Job drawing, mm, ordinate dimensions from the low corner. One solid piece. A direction names the side the tool comes from. Give positions to 0.01 mm unless a question says otherwise; leave off trailing zeros. Order: outer loops, then holes, each group sorted by start corner. A loop starts at its lowest first (then second) coordinate and runs counter-clockwise, first axis right, second up. Notation, with made-up numbers: (78.5, 26.25) - (90.5, 26.25) arc R12 ccw to (90.5, 33.25) - close; hole circle Ø10 at (89, 18.25). An arc over 180 degrees is marked (long way). Write each question's results on one line, items separated by ' | '. Start each with the question number.
1) Cut at C-C on y = 10. List the corners of the cut face in (x, z).
2) Drop flat-ended pins along their axis: pin 1 Ø7 at (x, y) = (10, 70) entering from -Z; pin 2 Ø17.5 at (y, z) = (18.5, 29) entering from -X; pin 3 Ø1.2 at (x, z) = (11.5, 3) entering from -Y; pin 4 Ø1.2 at (x, z) = (11, 1.5) entering from +Y. Give the stop position or say it passes through.
3) Cut at A-A on z = 29. List the corners of the cut face in (x, y), plus the area to 3 significant figures.
4) Tool access for the marked faces 1 and 2: list every direction of +Z, -Z, +X, -X, +Y, -Y with a clear straight run to the whole face (end or side of a thin tool).
5) Drill centre lines: line 1 along Z through (x, y) = (13, 130); line 2 along Y through (x, z) = (10, 7.5); line 3 along Y through (x, z) = (10.25, 15). Where is each one in solid material? Low to high. Write a range as from..to.
6) Cut at B-B on y = 70. List the corners of the cut face in (x, z).
7) Cut at D-D on y = 119.5. List the corners of the cut face in (x, z).
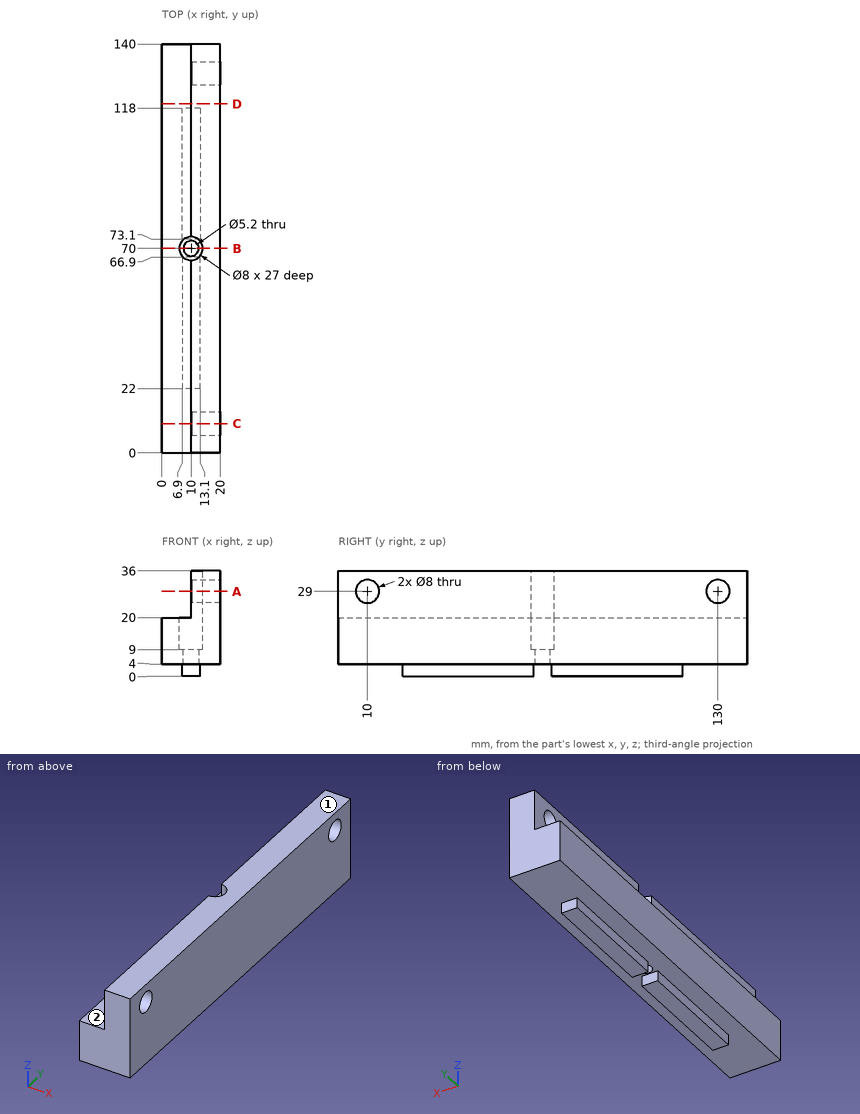
Results:
1) outline: (0, 4) - (20, 4) - (20, 25) - (10, 25) - (10, 20) - (0, 20) - close; (10, 33) - (20, 33) - (20, 36) - (10, 36) - close
2) pin 1: z = 0 | pin 2: x = 10 | pin 3: y = 22 | pin 4: y = 118
3) outline: (10, 0) - (20, 0) - (20, 6) - (10, 6) - close; (10, 14) - (20, 14) - (20, 126) - (10, 126) - (10, 74) arc R4 cw to (10, 66) - close; (10, 134) - (20, 134) - (20, 140) - (10, 140) - close | area: 1,210 mm^2
4) face 1: +Z, +X, -X, +Y, -Y | face 2: +Z, -X, +Y, -Y
5) line 1: 4..25, 33..36 | line 2: 0..67.4, 72.6..140 | line 3: 0..66.01, 73.99..140
6) outline: (0, 4) - (7.4, 4) - (7.4, 9) - (6, 9) - (6, 20) - (0, 20) - close; (12.6, 4) - (20, 4) - (20, 36) - (14, 36) - (14, 9) - (12.6, 9) - close
7) outline: (0, 4) - (20, 4) - (20, 36) - (10, 36) - (10, 20) - (0, 20) - close
